from build123d import *

# Parameters (mm, degrees)
SKETCH_1_R          = 1.5
SKETCH_1_W          = 9.7
SKETCH_1_H          = 1.95
EXTRUDE_3_DEPTH     = 3
CUT_EXTRUDE_1_DEPTH = 10


with BuildPart() as part:
    # Эскиз1 → Бобышка-Вытянуть3 (new body)
    with BuildSketch(Plane.XY):
        with BuildLine():
            Line((-88.837912602, -46.410254038), (-84.611415294, -53.730762114))
            Line((-84.611415294, -53.730762114), (-83.299663948, -56.002782092))
            ThreePointArc((-83.299663948, -56.002782092), (-81.478044872, -57.40055957), (-79.201587737, -57.100858303))
            Line((-79.201587737, -57.100858303), (-54.952876431, -43.100858303))
            ThreePointArc((-54.952876431, -43.100858303), (-52.676419295, -42.801157035), (-50.854800219, -44.198934514))
            Line((-50.854800219, -44.198934514), (-42.598076211, -58.5))
            ThreePointArc((-42.598076211, -58.5), (-41.5, -59.598076211), (-40, -60))
            Line((-40, -60), (40, -60))
            ThreePointArc((40, -60), (41.5, -59.598076211), (42.598076211, -58.5))
            Line((42.598076211, -58.5), (50.854800219, -44.198934514))
            ThreePointArc((50.854800219, -44.198934514), (52.676419295, -42.801157035), (54.952876431, -43.100858303))
            Line((54.952876431, -43.100858303), (79.201587737, -57.100858303))
            ThreePointArc((79.201587737, -57.100858303), (81.478044872, -57.40055957), (83.299663948, -56.002782092))
            Line((83.299663948, -56.002782092), (84.611415294, -53.730762114))
            Line((84.611415294, -53.730762114), (88.837912602, -46.410254038))
            Line((88.837912602, -46.410254038), (90.149663948, -44.13823406))
            ThreePointArc((90.149663948, -44.13823406), (90.449365215, -41.861776924), (89.051587737, -40.040157848))
            Line((89.051587737, -40.040157848), (64.802876431, -26.040157848))
            ThreePointArc((64.802876431, -26.040157848), (63.405098952, -24.218538772), (63.704800219, -21.942081637))
            Line((63.704800219, -21.942081637), (71.961524227, -7.641016151))
            ThreePointArc((71.961524227, -7.641016151), (72.363448016, -6.141016151), (71.961524227, -4.641016151))
            Line((71.961524227, -4.641016151), (31.961524227, 64.641016151))
            ThreePointArc((31.961524227, 64.641016151), (30.863448016, 65.739092363), (29.363448016, 66.141016151))
            Line((29.363448016, 66.141016151), (12.85, 66.141016151))
            ThreePointArc((12.85, 66.141016151), (10.728679656, 67.019695808), (9.85, 69.141016151))
            Line((9.85, 69.141016151), (9.85, 97.141016151))
            ThreePointArc((9.85, 97.141016151), (8.971320344, 99.262336495), (6.85, 100.141016151))
            Line((6.85, 100.141016151), (4.226497308, 100.141016151))
            Line((4.226497308, 100.141016151), (-4.226497308, 100.141016151))
            Line((-4.226497308, 100.141016151), (-6.85, 100.141016151))
            ThreePointArc((-6.85, 100.141016151), (-8.971320344, 99.262336495), (-9.85, 97.141016151))
            Line((-9.85, 97.141016151), (-9.85, 69.141016151))
            ThreePointArc((-9.85, 69.141016151), (-10.728679656, 67.019695808), (-12.85, 66.141016151))
            Line((-12.85, 66.141016151), (-29.363448016, 66.141016151))
            ThreePointArc((-29.363448016, 66.141016151), (-30.863448016, 65.739092363), (-31.961524227, 64.641016151))
            Line((-31.961524227, 64.641016151), (-71.961524227, -4.641016151))
            ThreePointArc((-71.961524227, -4.641016151), (-72.363448016, -6.141016151), (-71.961524227, -7.641016151))
            Line((-71.961524227, -7.641016151), (-63.704800219, -21.942081637))
            ThreePointArc((-63.704800219, -21.942081637), (-63.405098952, -24.218538772), (-64.802876431, -26.040157848))
            Line((-64.802876431, -26.040157848), (-89.051587737, -40.040157848))
            ThreePointArc((-89.051587737, -40.040157848), (-90.449365215, -41.861776924), (-90.149663948, -44.13823406))
            Line((-90.149663948, -44.13823406), (-88.837912602, -46.410254038))
        make_face()
        with Locations((-83.260562333, -48.070508076)):
            Circle(SKETCH_1_R, mode=Mode.SUBTRACT)
        with Locations(Location((83.260562333, -48.070508076, 0), (0, 0, 180))):
            Circle(SKETCH_1_R, mode=Mode.SUBTRACT)
        with Locations((0, 96.141016151)):
            Circle(SKETCH_1_R, mode=Mode.SUBTRACT)
        Polygon((-77.804473419, -50.520731284), (-82.654473419, -42.120284867), (-80.965723882, -41.145284867), (-76.115723882, -49.545731284), align=None, mode=Mode.SUBTRACT)
        Polygon((-71.309282891, -46.770731284), (-76.159282891, -38.370284867), (-74.470533354, -37.395284867), (-69.620533354, -45.795731284), align=None, mode=Mode.SUBTRACT)
        Polygon((69.620533354, -45.795731284), (74.470533354, -37.395284867), (76.159282891, -38.370284867), (71.309282891, -46.770731284), align=None, mode=Mode.SUBTRACT)
        Polygon((76.115723882, -49.545731284), (80.965723882, -41.145284867), (82.654473419, -42.120284867), (77.804473419, -50.520731284), align=None, mode=Mode.SUBTRACT)
        with Locations((0, 91.666016151)):
            Rectangle(SKETCH_1_W, SKETCH_1_H, mode=Mode.SUBTRACT)
        with Locations((0, 84.166016151)):
            Rectangle(SKETCH_1_W, SKETCH_1_H, mode=Mode.SUBTRACT)
    extrude(amount=EXTRUDE_3_DEPTH)

    # Эскиз2 → Вырез-Вытянуть1 (cut)
    with BuildSketch(Plane.XY.offset(3)):
        with BuildLine():
            Line((28.29016319, -46), (53.982250169, -1.5))
            ThreePointArc((53.982250169, -1.5), (54.384173958, 0), (53.982250169, 1.5))
            Line((53.982250169, 1.5), (28.29016319, 46))
            ThreePointArc((28.29016319, 46), (27.192086979, 47.098076211), (25.692086979, 47.5))
            Line((25.692086979, 47.5), (-25.692086979, 47.5))
            ThreePointArc((-25.692086979, 47.5), (-27.192086979, 47.098076211), (-28.29016319, 46))
            Line((-28.29016319, 46), (-53.982250169, 1.5))
            ThreePointArc((-53.982250169, 1.5), (-54.384173958, 0), (-53.982250169, -1.5))
            Line((-53.982250169, -1.5), (-28.29016319, -46))
            ThreePointArc((-28.29016319, -46), (-27.192086979, -47.098076211), (-25.692086979, -47.5))
            Line((-25.692086979, -47.5), (25.692086979, -47.5))
            ThreePointArc((25.692086979, -47.5), (27.192086979, -47.098076211), (28.29016319, -46))
        make_face()
    extrude(amount=-CUT_EXTRUDE_1_DEPTH, mode=Mode.SUBTRACT)


solid = part.part
Could you check a few things on this model? Use its own coordinates, in mm. A direction names the side the tool comes from. Give positions to 0.01 mm unless a question says otherwise; leave off trailing zeros. Order: outer loops, then holes, each group sorted by start corner. A loop starts at its lowest first (then second) coordinate and runs counter-clockwise, first axis right, second up.
1. Will these pins go through, and if not, where does the flat tip stop? P1, Ø1.5, axis at y = 84.5, z = 1.5, coming from the -X side; P2, Ø0.6, axis at y = 91.5, z = 1, coming from the +X side; P3, Ø1.6, axis at y = 84.5, z = 2, coming from the +X side.
2. Suppose I cut it at C-C (z = 0.45). Give the number of separate pieces and of enclosed holes in the cut face, plus the area to 3 significant figures.
3. Suppose I cut it at A-A (x = 21). List the corners of the cut face in (y, z) for me, plus the area to 3 significant figures.
4. Suppose I cut it at B-B (y = -24). List the corners of the cut face in (x, z) for me, plus the area to 3 significant figures.
5. I need wall thicknesses on L1, parallel to Y at x = 20, z = 1.1; L2, parallel to X at y = 89.5, z = 2.85; L3, parallel to X at y = -14.5, z = 2.2. Which ranges of each line are inside material? Lowest first, please.
6. We'd pull the mould along X, two halves only. Please class faces 4 (the flat face through (47, 15, 0)), 5 (the flat face through (-51.682, 30.485, 1.479)), 6 (the flat face through (78.51, -45.4, 1.48)): pulls with the +X half, pulls with the -X half, needs draft (parallel to the pull), parting line crosses it, or undercut.
7. For faces 1 (the flat face through (-76.757, -32.942, 1.479)), 2 (the flat face through (77.1, -33.14, 1.48)), 3 (the flat face through (-80.196, -46.379, 1.479)), which set-ups out of +Z, -Z, +X, -X, +Y, -Y let a thin tool reach every point of the face, with its end or its side?
Solved:
1. P1: stops at x = -9.85
1. P2: stops at x = 9.85
1. P3: stops at x = 9.85
2. separate pieces: 1
2. enclosed holes: 10
2. area: 7,740 mm2
3. outline: (-60, 0) - (-47.5, 0) - (-47.5, 3) - (-60, 3) - close; (47.5, 0) - (66.14, 0) - (66.14, 3) - (47.5, 3) - close
3. area: 93.4 mm2
4. outline: (-63.36, 0) - (-40.99, 0) - (-40.99, 3) - (-63.36, 3) - close; (40.99, 0) - (63.36, 0) - (63.36, 3) - (40.99, 3) - close
4. area: 134 mm2
5. L1: y = -60 to -47.5, 47.5 to 66.14
5. L2: x = -9.85 to 9.85
5. L3: x = -68 to -46.48, 46.48 to 68
6. face 4: needs draft
6. face 5: pulls with the -X half
6. face 6: undercut
7. face 1: +Z, -Z, -X
7. face 2: +Z, -Z, +X
7. face 3: +Z, -Z
